Geometry: final body of the model. Coordinates: model frame, mm. A direction names the side the tool comes from. Give positions to 0.01 mm unless a question says otherwise; leave off trailing zeros. Write each loop counter-clockwise with the first axis right and the second up, starting at its lowest first coordinate (ties: lowest second). Pieces come first, ordered by that corner, then holes. Notation, with made-up numbers: M 16,-18 L 72,-18 A16 cw 72,1 Z; hole C 5.25,-21 d10. An arc over 180 degrees is marked long. One line per question, with ' | ' between items.
from build123d import *


with BuildPart() as f3:
    # F0 (on Top) → F3 section 0
    with BuildSketch(Plane.XY, mode=Mode.PRIVATE) as f3_s0:
        Polygon((-47.688171, 47.806267), (-67.121834, 9.70584), (-72.229996, -52.108184), (-39.03887, -9.052839), (-9.768937, -73.99904), (15.477421, -9.052839), (71.840197, -37.801471), (34.815956, 17.355996), (50.347548, 47.806267), (9.988855, 21.649893), (-9.729384, 47.806267), (-31.556629, 21.649893), align=None)
    loft([f3_s0.sketch, Vertex(8.825648, -51.505208, 254)])


solid = f3.part
(1) First-contact query: P1, Ø10, axis at y = -56.5, z = 77, coming from the +X side; P2, Ø2, axis at y = -2.5, z = 100.5, coming from the -X side; P3, Ø10, axis at x = -5.5, z = 42, coming from the +Y side. Flat tips, straight axial feed; report the tip coordinate or a pass-through.
Working result:
P1: stops at x = 1.97 | P2: stops at x = -31.61 | P3: stops at y = 33.25
(2) Set-up query: faces 1 (the face through (-47.296, -29.53, 72.334)), 2 (the face through (4.22, 5.61, 80.56)), 3 (the face through (31.717, -30.392, 72.334)). Return all of +Z, -Z, +X, -X, +Y, -Y with unobstructed straight access to the full face (end or side cutting, diameter ignored); none if empty.
Working result:
face 1: +Z, -X, +Y | face 2: +Z, +Y | face 3: -Z, -Y
(3) Cut plane C-C, the plane x = 45. Return loops of the section in (y, z), then the cut area to 3 significant figures.
Working result:
outline: M -43.64,108.19 L -24.11,0 L 2.18,0 Z; M 35.02,32.71 L 37.32,0 L 44.34,0 Z | area: 1,540 mm^2
(4) Draft query along Z for faces 4 (the face through (-37.8, -37.2, 72.3)), 5 (the face through (20.957, 5.796, 80.556)), 6 (the face through (-11.9, -44.03, 100.56)), 7 (the face through (-10, 3, 0)). Return one class per face: released by +Z, released by -Z, zero draft, split by the parting line, or undercut.
Working result:
face 4: undercut | face 5: released by +Z | face 6: undercut | face 7: released by -Z
(5) Cut plane D-D, the plane x = -28. Return loops of the section in (y, z) (3 decimals), then the cut area to 3 significant figures.
Working result:
outline: M -51.779,138.601 L -18.844,58.579 L -33.547,0 L 25.912,0 L 15.207,22.371 L 13.208,88.488 L -21.825,130.84 Z | area: 5,290 mm^2
(6) Material intervals for L1, parallel to X at y = -24, z = 12; L2, parallel to X at y = -33, z = 16; L3, parallel to X at y = -56.5, z = 133, sorted ascending. Write a range as [from, to].
Working result:
L1: x = [-66.08, -46.75], [-30.95, 10.13], [40.54, 59.16] | L2: x = [-65.55, -52.42], [-26.44, 6.79], [56.76, 64.07] | L3: x = [-2.61, 2.19]
(7) Cut plane A-A, the plane y = 26.5. Return loops of the section in (x, z), then the cut area to 3 significant figures.
Working result:
outline: M -58.56,0 L -34.55,0 L -35.56,54.49 Z; M -27.51,0 L 6.33,0 L -5.75,54.49 Z; M 17.47,0 L 39.48,0 L 41.44,54.49 Z | area: 2,180 mm^2
(8) Cut plane B-B, the plane z = 195. Return loops of the section in (x, y), then the cut area to 3 significant figures.
Working result:
outline: M -10,-51.65 L -2.29,-41.64 L 4.51,-56.73 L 10.37,-41.64 L 23.46,-48.32 L 14.86,-35.51 L 18.47,-28.44 L 9.1,-34.51 L 4.52,-28.44 L -0.55,-34.51 L -4.3,-28.44 L -8.82,-37.29 Z | area: 408 mm^2
